Model file for the job. Use its own axes, mm. A direction names the side the tool comes from. Round coordinates to 2 decimals unless told otherwise and drop trailing zeros. Write each loop counter-clockwise with the first axis right and the second up, starting at its lowest first coordinate (ties: lowest second). Pieces come first, ordered by that corner, then holes. Notation, with made-up numbers: (-32.75, -21.75) - (22.25, -21.75) arc R29 cw to (22.25, -0.75) - close; hole circle Ø1 at (9.5, 20). An arc over 180 degrees is marked (long way). One line per item, written item: value.
from build123d import *


with BuildPart() as part:
    # Sketch1 → Revolve1 (revolve)
    with BuildSketch(Plane.XY):
        with BuildLine():
            Line((12.7, -6.150685179), (6.455964927, 3.675363757))
            Line((6.455964927, 3.675363757), (4.742541645, 3.675363757))
            ThreePointArc((4.742541645, 3.675363757), (5.387586776, -2.640815921), (0, -6))
            Line((0, -6), (0, -9.059401987))
            Line((0, -9.059401987), (11.244226909, -9.059401987))
            ThreePointArc((11.244226909, -9.059401987), (11.5977803, -8.912955378), (11.744226909, -8.559401987))
            Line((11.744226909, -8.559401987), (11.744226909, -8.340026624))
            Line((11.744226909, -8.340026624), (12.7, -8.340026624))
            Line((12.7, -8.340026624), (12.7, -6.150685179))
        make_face()
    revolve(axis=Axis((0, 0, 0), (0, -1, 0)))


solid = part.part
1. Band-saw the part on D-D on y = -1. Write the cut outline in (x, z).
Report:
outline: circle Ø18.85 at (0, 0); hole circle Ø11.83 at (0, 0)
2. Band-saw the part on A-A on z = 0. Write the cut outline in (x, y).
Report:
outline: (-12.7, -8.34) - (-11.74, -8.34) - (-11.74, -8.56) arc R0.5 ccw to (-11.24, -9.06) - (11.24, -9.06) arc R0.5 ccw to (11.74, -8.56) - (11.74, -8.34) - (12.7, -8.34) - (12.7, -6.15) - (6.46, 3.68) - (4.74, 3.68) arc R6 cw (long way) to (-4.74, 3.68) - (-6.46, 3.68) - (-12.7, -6.15) - close
3. Band-saw the part on B-B on x = 0. Write the cut outline in (y, z).
Report:
outline: (-9.06, -11.24) arc R0.5 ccw to (-8.56, -11.74) - (-8.34, -11.74) - (-8.34, -12.7) - (-6.15, -12.7) - (3.68, -6.46) - (3.68, -4.74) arc R6 cw (long way) to (3.68, 4.74) - (3.68, 6.46) - (-6.15, 12.7) - (-8.34, 12.7) - (-8.34, 11.74) - (-8.56, 11.74) arc R0.5 ccw to (-9.06, 11.24) - close
4. Wall check: probe 1 along X at (y, z) = (-3.5, -2.25); probe 2 along Y at (x, z) = (-4.25, -2.5); probe 3 along Z at (x, y) = (-3.25, -2). Give the ranges that are in metal, low to high. Write a range as [from, to].
Report:
probe 1: [-10.78, -4.32], [4.32, 10.78]
probe 2: [-9.06, -3.42], [3.42, 3.68]
probe 3: [-9.52, -4.63], [4.63, 9.52]
5. Tool access for faces 1 (the face through (0, -9.059, 0)), 2 (the face through (-7.5, -8.34, -9.3)): list every direction of +Z, -Z, +X, -X, +Y, -Y with a clear straight run to the whole face (end or side of a thin tool).
Report:
face 1: +Z, -Z, +X, -X, -Y
face 2: -Y
6. Mould opens along Z. For faces 3 (the face through (0, 3.675, 5)), 4 (the face through (-2.75, -7.23, -12.4)) say: released by +Z, released by -Z, zero draft, split by the parting line, or undercut.
Report:
face 3: zero draft
face 4: split by the parting line
7. Band-saw the part on C-C on y = 1. Write the cut outline in (x, z), plus the area to 3 significant figures.
Report:
outline: circle Ø16.31 at (0, 0); hole circle Ø11.83 at (0, 0)
area: 99.0 mm²
8. Drop flat-ended pins along their axis: pin 1 (1 mm diameter, centred on x = 9, z = -6, fed in from +Y); pin 2 (1 mm diameter, centred on y = 1.5, z = 6, fed in from +X); pin 3 (4 mm diameter, centred on x = -5, y = -3, fed in from -Z). Give the stop position or say it passes through.
Report:
pin 1: y = -2.4
pin 2: x = 5.76
pin 3: z = -11.1
